Autodesk Inventor part; units mm, degrees
ref_plane "YZ Plane" through (0, 0, 0) normal (1, 0, 0) x (0, 1, 0)
ref_plane "XZ Plane" through (0, 0, 0) normal (0, 1, 0) x (-1, 0, 0)
ref_plane "XY Plane" through (0, 0, 0) normal (0, 0, 1) x (1, 0, 0)
sketch "Sketch1" plane through (0, 0, 0) normal (0, 1, 0) x (-1, 0, 0)
  circle A0 centre (0, 0) radius 14.732
  dimension "d0" = 29.464
extrude "Extrusion1" add sketch "Sketch1" along normal blind 7.9248
sketch "Sketch2" plane through (0, 7.9248, 0) normal (0, 1, 0) x (1, 0, 0)
  circle A0 centre (0, 0) radius 14.732
  circle A1 centre (0, 0) radius 13.9065
  dimension "d3" = 27.813
extrude "Extrusion2" add sketch "Sketch2" along normal blind 13.97 contours A1
sketch "Sketch4" plane through (0, 7.9248, 0) normal (0, 1, 0) x (1, 0, 0)
  circle A0 centre (0, 0) radius 13.9065
  circle A1 centre (0, 0) radius 14.732
  circle A2 centre (0, 0) radius 13.9065
  circle A3 centre (0, 0) radius 14.732
  line L0 (-13.905, 0.2046) -> (-13.0794, 0.2046) construction
  line L1 (-13.9052, 0.1905) -> (-14.7308, 0.1905)
  line L2 (-13.9052, 0.1905) -> (-13.0796, 0.1905) construction
  line L3 (-13.9052, -0.1905) -> (-14.7308, -0.1905)
  line L4 (-13.9052, -0.1905) -> (-13.0796, -0.1905) construction
  line L5 (-13.9052, 0.1905) -> (14.7308, 0.1896)
  line L6 (-13.9052, -0.1905) -> (14.7307, -0.1927)
  dimension "d7" = 180
  dimension "d8" = 180
extrude "Extrusion3" add sketch "Sketch4" along normal blind 12.7 contours L5 A0 L6 | A0 L3 A1 L1 | L5 A1 L6 A0
chamfer "Chamfer1" distance 0.508 angle 45 1 edges at (14.732, 20.6248, 0.0015)
chamfer "Chamfer2" distance 0.508 angle 45 1 edges at (-14.732, 20.6248, 0)
fillet "Fillet1" radius 1.27 1 edges at (-13.9065, 21.8948, 0)
fillet "Fillet2" radius 0.508 1 edges at (0.0004, 7.9248, -14.732)
sketch "Sketch5" plane through (0, 21.8948, 0) normal (0, 1, 0) x (1, 0, 0)
  circle A0 centre (0, 0) radius 12.6365
  circle A1 centre (0, 0) radius 7.9375
  dimension "d19" = 15.875
extrude "Extrusion4" cut sketch "Sketch5" against normal blind 25.4 contours A1
sketch "Sketch6" plane through (0, 0, 0) normal (0, -1, 0) x (1, 0, 0)
  circle A0 centre (0, 0) radius 7.9375
  circle A1 centre (0, 0) radius 14.732
  circle A2 centre (0, 0) radius 7.9375
  circle A3 centre (0, 0) radius 1.5
  dimension "d22" = 3
extrude "Extrusion5" add sketch "Sketch6" against normal blind 21.8948 contours A0
properties part number "Pipe Cap 3 - Kapton Tape"
Could you check a few things on this model? Use its own coordinates, in mm. A direction names the side the tool comes from. Round coordinates to 2 decimals unless told otherwise and drop trailing zeros. Write each loop counter-clockwise with the first axis right and the second up, starting at its lowest first coordinate (ties: lowest second). Pieces come first, ordered by that corner, then holes. Notation, with made-up numbers: (83, -27.75) -> (131, -27.75) arc R20 ccw to (131, -2.75) -> close; hole circle Ø1 at (-12.5, -4). An arc over 180 degrees is marked (long way). Use a Markdown table: item, result.
1. Which directions (+Z, -Z, +X, -X, +Y, -Y) give clear straight access to the entire face, cutting with the end or side of a thin tool? Please do faces 1 (the face through (2, 7.925, 14)), 2 (the face through (3, 0, 0)), 3 (the face through (-14.3, 14.2, 0.19)).
Answer key:
| item | result |
|---|---|
| face 1 | +Z, +Y |
| face 2 | +Z, -Z, +X, -X, -Y |
| face 3 | +Z, -X, +Y |
2. If we section it at A-A (x = 0): List the corners of the cut face in (y, z) for me, then the cut area to 3 significant figures.
Answer key:
| item | result |
|---|---|
| outline | (0, -14.73) -> (7.42, -14.73) arc R0.51 ccw to (7.92, -14.22) -> (7.92, -13.91) -> (20.62, -13.91) arc R1.27 ccw to (21.89, -12.64) -> (21.89, -1.5) -> (0, -1.5) -> close; (0, 1.5) -> (21.89, 1.5) -> (21.89, 12.64) arc R1.27 ccw to (20.62, 13.91) -> (7.92, 13.91) -> (7.92, 14.73) -> (0, 14.73) -> close |
| area | 556 mm^2 |
3. Please list where these lines run through material, in increasing order: probe 1 along Z at (x, y) = (0, 12.5); probe 2 along Z at (x, y) = (0, 5.5); probe 3 along Z at (x, y) = (-9, 4.5).
Answer key:
| item | result |
|---|---|
| probe 1 | z = -13.91 to -1.5, 1.5 to 13.91 |
| probe 2 | z = -14.73 to -1.5, 1.5 to 14.73 |
| probe 3 | z = -11.66 to 11.66 |
4. If we section it at C-C (y = 5.75): List the corners of the cut face in (x, z) for me, then the cut area to 3 significant figures.
Answer key:
| item | result |
|---|---|
| outline | circle Ø29.46 at (0, 0); hole circle Ø3 at (0, 0) |
| area | 675 mm^2 |
5. For pin 1 Ø0.9 at (x, y) = (-14.5, 11.5) entering from -Z; pin 2 Ø0.9 at (x, y) = (14.5, 11.5) entering from +Z; pin 3 Ø10 at (y, z) = (15.5, 9.5) entering from -X, each with a flat end and sliding along its axis, tell me the tip position at first contact or that it passes through.
Answer key:
| item | result |
|---|---|
| pin 1 | stops at z = -0.19 |
| pin 2 | stops at z = 0.19 |
| pin 3 | stops at x = -13.16 |
6. We'd pull the mould along Z, two halves only. Please class faces 4 (the face through (3, 21.895, 0)), 5 (the face through (-1.5, 10.79, 0.07)), 6 (the face through (-14.3, 13.9, -0.19)), 7 (the face through (-11.036, 14.186, -8.462)): +Z half, -Z half, draft (parallel to the pull), parting line (faces both ways), or undercut.
Answer key:
| item | result |
|---|---|
| face 4 | draft |
| face 5 | undercut |
| face 6 | -Z half |
| face 7 | parting line |
